Verification items for the finished model (mm, model axes). Face numbers are marked on the shaded views. Round coordinates to 2 decimals unless told otherwise and drop trailing zeros. Write each loop counter-clockwise with the first axis right and the second up, starting at its lowest first coordinate (ties: lowest second). Pieces come first, ordered by that corner, then holes.
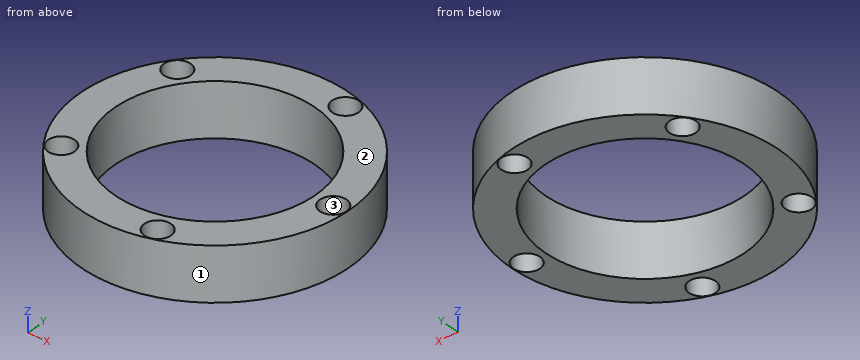
from build123d import *

# Parameters (mm, degrees)
SKETCH_1_R          = 12
SKETCH_1_R_2        = 1
EXTRUDE_1_DEPTH     = 2
SKETCH_3_R          = 1
EXTRUDE_2_DEPTH     = 12
SKETCH_4_R          = 7
CUT_EXTRUDE_1_DEPTH = 12
SKETCH_6_R          = 12
SKETCH_6_R_2        = 11.5
CUT_EXTRUDE_2_DEPTH = 4
SKETCH_8_R          = 11.5
SKETCH_8_R_2        = 7
EXTRUDE_4_DEPTH     = 2
SKETCH_9_R          = 7.5
CUT_EXTRUDE_3_DEPTH = 4
SKETCH_12_R         = 1
CUT_EXTRUDE_4_DEPTH = 20
SKETCH_13_R         = 11.5
SKETCH_13_R_2       = 10.05
CUT_EXTRUDE_5_DEPTH = 10


with BuildPart() as part:
    # 草图1 → 凸台-拉伸1 (new body)
    with BuildSketch(Plane.XY):
        Circle(SKETCH_1_R)
        with Locations((9, 0)):
            Circle(SKETCH_1_R_2, mode=Mode.SUBTRACT)
        with Locations((2.781152949, -8.559508647)):
            Circle(SKETCH_1_R_2, mode=Mode.SUBTRACT)
        with Locations((-7.281152949, -5.290067271)):
            Circle(SKETCH_1_R_2, mode=Mode.SUBTRACT)
        with Locations((-7.281152949, 5.290067271)):
            Circle(SKETCH_1_R_2, mode=Mode.SUBTRACT)
        with Locations((2.781152949, 8.559508647)):
            Circle(SKETCH_1_R_2, mode=Mode.SUBTRACT)
    extrude(amount=EXTRUDE_1_DEPTH)

    # 草图3 → 凸台-拉伸2 (add)
    with BuildSketch(Plane.XY.offset(2)):
        with Locations((9, 0)):
            Circle(SKETCH_3_R)
        with Locations((2.781152949, -8.559508647)):
            Circle(SKETCH_3_R)
        with Locations((-7.281152949, -5.290067271)):
            Circle(SKETCH_3_R)
        with Locations((-7.281152949, 5.290067271)):
            Circle(SKETCH_3_R)
        with Locations((2.781152949, 8.559508647)):
            Circle(SKETCH_3_R)
    extrude(amount=-EXTRUDE_2_DEPTH)

    # 草图4 → 切除-拉伸1 (cut)
    with BuildSketch(Plane(origin=(0, 0, 0), x_dir=(-1, 0, 0), z_dir=(0, 0, -1))):
        Circle(SKETCH_4_R)
    extrude(amount=-CUT_EXTRUDE_1_DEPTH, mode=Mode.SUBTRACT)

    # 草图6 → 切除-拉伸2 (cut)
    with BuildSketch(Plane(origin=(0, 0, 0), x_dir=(-1, 0, 0), z_dir=(0, 0, -1))):
        Circle(SKETCH_6_R)
        Circle(SKETCH_6_R_2, mode=Mode.SUBTRACT)
    extrude(amount=-CUT_EXTRUDE_2_DEPTH, mode=Mode.SUBTRACT)

    # 草图8 → 凸台-拉伸4 (add)
    with BuildSketch(Plane.XY.offset(2)):
        Circle(SKETCH_8_R)
        Circle(SKETCH_8_R_2, mode=Mode.SUBTRACT)
    extrude(amount=EXTRUDE_4_DEPTH)

    # 草图9 → 切除-拉伸3 (cut)
    with BuildSketch(Plane(origin=(0, 0, 0), x_dir=(-1, 0, 0), z_dir=(0, 0, -1))):
        Circle(SKETCH_9_R)
    extrude(amount=-CUT_EXTRUDE_3_DEPTH, mode=Mode.SUBTRACT)

    # 草图12 → 切除-拉伸4 (cut)
    with BuildSketch(Plane(origin=(0, 0, -10), x_dir=(-1, 0, 0), z_dir=(0, 0, -1))):
        with Locations((-2.781152949, -8.559508647)):
            Circle(SKETCH_12_R)
        with Locations((7.281152949, 5.290067271)):
            Circle(SKETCH_12_R)
        with Locations((-2.781152949, 8.559508647)):
            Circle(SKETCH_12_R)
        with Locations((-9, 0)):
            Circle(SKETCH_12_R)
        with Locations((7.281152949, -5.290067271)):
            Circle(SKETCH_12_R)
    extrude(amount=-CUT_EXTRUDE_4_DEPTH, mode=Mode.SUBTRACT)

    # 草图13 → 切除-拉伸5 (cut)
    with BuildSketch(Plane.XY.offset(4)):
        Circle(SKETCH_13_R)
        Circle(SKETCH_13_R_2, mode=Mode.SUBTRACT)
    extrude(amount=-CUT_EXTRUDE_5_DEPTH, mode=Mode.SUBTRACT)


solid = part.part
Q1. Material ranges on line 1 along Y through (x, z) = (0, 2.6); line 2 along X through (y, z) = (0.75, 2.6); line 3 along X through (y, z) = (-5, 3.3), recorded low to high.
Recorded:
line 1: y = -10.05 to -7.5, 7.5 to 10.05
line 2: x = -10.02 to -7.46, 7.46 to 8.34, 9.66 to 10.02
line 3: x = -8.72 to -8.24, -6.32 to -5.59, 5.59 to 8.72
Q2. Release check for a two-part mould opening along Y. For the marked faces 1, 2 and 3 record: released by +Y, released by -Y, zero draft, split by the parting line, or undercut.
Recorded:
face 1: split by the parting line
face 2: zero draft
face 3: undercut
Q3. Sectioned sample at A-A (x = 0). Enter the section's corners in (y, z), plus the area to 3 significant figures.
Recorded:
outline: (-10.05, 0) - (-7.5, 0) - (-7.5, 4) - (-10.05, 4) - close; (7.5, 0) - (10.05, 0) - (10.05, 4) - (7.5, 4) - close
area: 20.4 mm2
Q4. Depth check by flat-ended pin: P1, Ø1.5, axis at x = -5, z = 3, coming from the +Y side. Enter the tip coordinate at first touch or a pass-through.
Recorded:
P1: stops at y = 9.11
Q5. Sectioned sample at D-D (z = 3.2). Enter the section's corners in (x, y).
Recorded:
outline: circle Ø20.1 at (0, 0); hole circle Ø2 at (-7.28, -5.29); hole circle Ø2 at (-7.28, 5.29); hole circle Ø15 at (0, 0); hole circle Ø2 at (2.78, -8.56); hole circle Ø2 at (2.78, 8.56); hole circle Ø2 at (9, 0)
Q6. Sectioned sample at C-C (y = 3.5). Enter the section's corners in (x, z), plus the area to 3 significant figures.
Recorded:
outline: (-9.42, 0) - (-6.63, 0) - (-6.63, 4) - (-9.42, 4) - close; (6.63, 0) - (9.42, 0) - (9.42, 4) - (6.63, 4) - close
area: 22.3 mm2
Q7. Sectioned sample at B-B (y = 0). Enter the section's corners in (x, z).
Recorded:
outline: (-10.05, 0) - (-7.5, 0) - (-7.5, 4) - (-10.05, 4) - close; (7.5, 0) - (8, 0) - (8, 4) - (7.5, 4) - close; (10, 0) - (10.05, 0) - (10.05, 4) - (10, 4) - close
